from build123d import *

# Parameters (mm, degrees)
SKETCH1_W           = 128.5
SKETCH1_H           = 160
BOSS_EXTRUDE1_DEPTH = 10
SKETCH6_W           = 6
SKETCH6_H           = 10
BOSS_EXTRUDE2_DEPTH = 10


with BuildPart() as part:
    # Sketch1 → Boss-Extrude1 (new body)
    with BuildSketch(Plane(origin=(0, 0, 0), x_dir=(1, 0, 0), z_dir=(0, 1, 0))):
        Rectangle(SKETCH1_W, SKETCH1_H)
    extrude(amount=BOSS_EXTRUDE1_DEPTH)

    # Sweep1: sweep along a path in Sketch4
    with BuildLine(Plane(origin=(64.25, 0, 0), x_dir=(0, 0, -1), z_dir=(1, 0, 0))) as sweep1_path:
        Line((-80, 10), (-37.738173826, 100.630778704))
    # Sketch2 → Sweep1 (sweep)
    with BuildSketch(Plane(origin=(0, 10, 0), x_dir=(1, 0, 0), z_dir=(0, 1, 0))):
        Polygon((-64.25, -80), (64.25, -80), (64.25, -67), (-64.25, -67), (-64.25, -72), (62.25, -72), (62.25, -75), (-64.25, -75), align=None)
    sweep(path=sweep1_path.line)

    # Sketch6 → Boss-Extrude2 (add)
    with BuildSketch(Plane(origin=(0, 10, 0), x_dir=(1, 0, 0), z_dir=(0, 1, 0))):
        with Locations((-61.25, 75)):
            Rectangle(SKETCH6_W, SKETCH6_H)
        with Locations((-61.25, -19.738173826)):
            Rectangle(SKETCH6_W, SKETCH6_H)
        with Locations((61.25, 75)):
            Rectangle(SKETCH6_W, SKETCH6_H)
        with Locations((61.25, -19.738173826)):
            Rectangle(SKETCH6_W, SKETCH6_H)
    extrude(amount=BOSS_EXTRUDE2_DEPTH)


solid = part.part
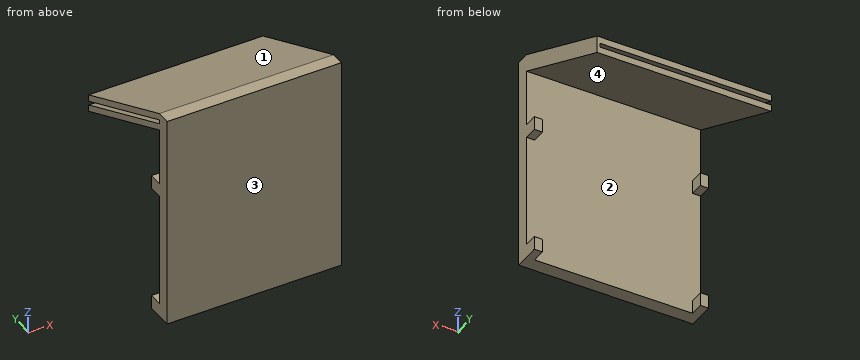
Part model, mm, in its own coordinate system. Face numbers are marked on the shaded views. Give positions to 0.01 mm unless a question says otherwise; leave off trailing zeros. Write each loop counter-clockwise with the first axis right and the second up, starting at its lowest first coordinate (ties: lowest second). Pieces come first, ordered by that corner, then holes.
1) Cut at A-A on z = 63. Write the cut outline in (x, y).
Resolved:
outline: (-64.25, 0) - (64.25, 0) - (64.25, 10) - (-64.25, 10) - close; (-64.25, 18.58) - (64.25, 18.58) - (64.25, 46.46) - (-64.25, 46.46) - (-64.25, 35.73) - (62.25, 35.73) - (62.25, 29.3) - (-64.25, 29.3) - close
2) Two-plate mould, pull along Y, no slides. Class the marked faces 1, 2, 3 and 4: released by +Y, released by -Y, zero draft, split by the parting line, or undercut.
Resolved:
face 1: released by +Y
face 2: undercut
face 3: released by -Y
face 4: undercut
3) Cut at D-D on z = -1.5. Write the cut outline in (x, y), then the cut area to 4 significant figures.
Resolved:
outline: (-64.25, 0) - (64.25, 0) - (64.25, 10) - (-64.25, 10) - close
area: 1,285 mm2
4) Cut at C-C on y = 36. Write the cut outline in (x, z).
Resolved:
outline: (-64.25, 54.88) - (64.25, 54.88) - (64.25, 67.88) - (-64.25, 67.88) - (-64.25, 62.88) - (62.25, 62.88) - (62.25, 59.88) - (-64.25, 59.88) - close
5) Cut at B-B on x = 52. Write the cut outline in (y, z), then the cut area to 3 significant figures.
Resolved:
outline: (0, -80) - (10, -80) - (10, 67) - (100.63, 24.74) - (100.63, 29.74) - (10, 72) - (10, 75) - (100.63, 32.74) - (100.63, 37.74) - (10, 80) - (0, 80) - close
area: 2,510 mm2
6) Pin check, flat tips, straight feed: pin 1 (1 mm diameter, centred on x = -7, y = 56, fed in from -Z); pin 2 (10 mm diameter, centred on x = 43, z = -51, fed in from -Y); pin 3 (6.5 mm diameter, centred on x = -60, z = -75, fed in from +Y); pin 4 (3 mm diameter, centred on x = -61, y = 13.5, fed in from +Z). Stop position of each tip, or through.
Resolved:
pin 1: stops at z = 45.32
pin 2: stops at y = 0
pin 3: stops at y = 20
pin 4: stops at z = 79.07
7) Probe L1, parallel to Y at x = -40.5, z = 37; L2, parallel to Y at x = 32.5, z = -31.5; L3, parallel to Z at x = 19, y = 44. List the from-to ranges inside material, lowest first.
Resolved:
L1: y = 0 to 10, 74.34 to 85.06, 91.49 to 100.63
L2: y = 0 to 10
L3: z = 51.15 to 56.15, 59.15 to 64.15
